Input: dimensioned drawing with shaded views. Units: mm. Origin: part minimum x, y, z. A direction names the side the tool comes from. Give positions to 0.01 mm unless a question says otherwise; leave off trailing zeros. Write each loop counter-clockwise with the first axis right and the second up, starting at its lowest first coordinate (ties: lowest second). Pieces come first, ordered by that corner, then holes.
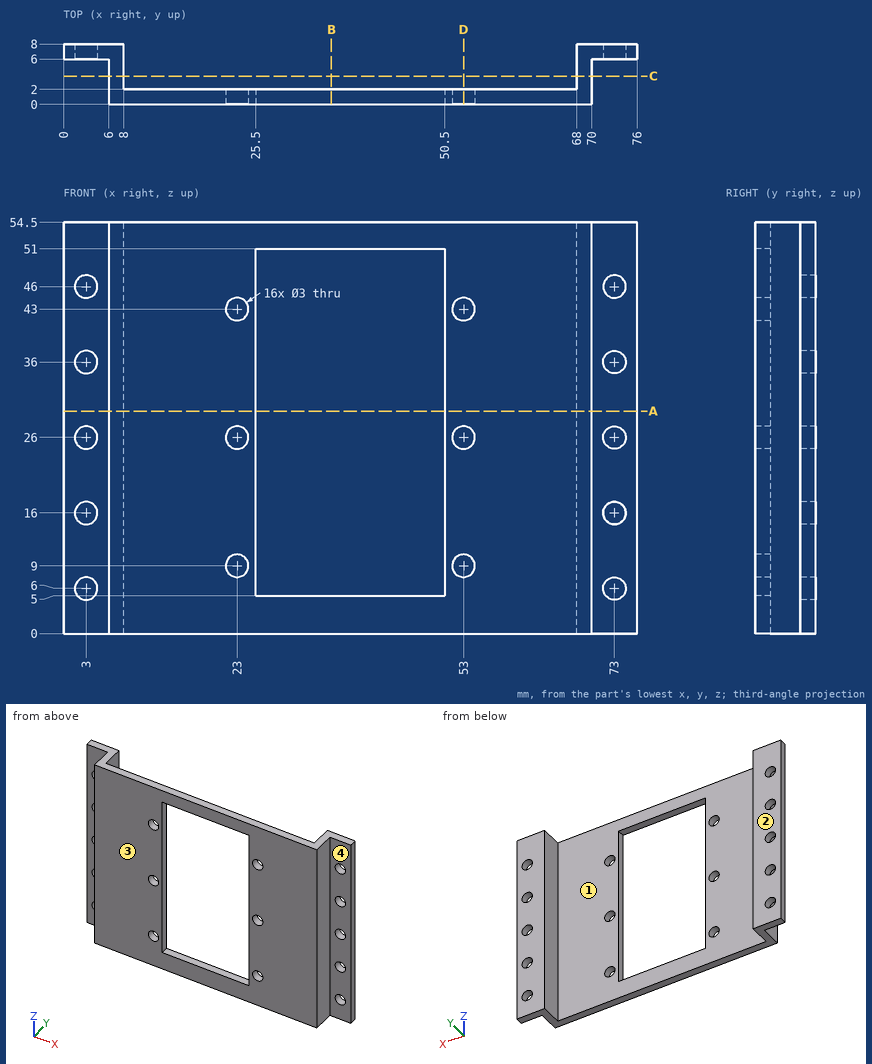
Item 1: Section A-A, the plane z = 29.5. Return the cut outline in (x, y), plus the area to 3 significant figures.
Found:
outline: (0, 6) - (6, 6) - (6, 0) - (25.5, 0) - (25.5, 2) - (8, 2) - (8, 8) - (0, 8) - close; (50.5, 0) - (70, 0) - (70, 6) - (76, 6) - (76, 8) - (68, 8) - (68, 2) - (50.5, 2) - close
area: 126 mm2
Item 2: Section C-C, the plane y = 3.75. Return the cut outline in (x, z).
Found:
outline: (6, 0) - (8, 0) - (8, 54.5) - (6, 54.5) - close; (68, 0) - (70, 0) - (70, 54.5) - (68, 54.5) - close
Item 3: Section B-B, the plane x = 35.5. Return the cut outline in (y, z).
Found:
outline: (0, 0) - (2, 0) - (2, 5) - (0, 5) - close; (0, 51) - (2, 51) - (2, 54.5) - (0, 54.5) - close
Item 4: Section D-D, the plane x = 53. Return the cut outline in (y, z), plus the area to 3 significant figures.
Found:
outline: (0, 0) - (2, 0) - (2, 7.5) - (0, 7.5) - close; (0, 10.5) - (2, 10.5) - (2, 24.5) - (0, 24.5) - close; (0, 27.5) - (2, 27.5) - (2, 41.5) - (0, 41.5) - close; (0, 44.5) - (2, 44.5) - (2, 54.5) - (0, 54.5) - close
area: 91.0 mm2
Item 5: Pin query (flat end, axial travel): pin 1 Ø2 at (y, z) = (5.5, 24) entering from +X; pin 2 Ø5 at (x, z) = (3, 21.5) entering from -Y; pin 3 Ø6 at (x, z) = (61.5, 23) entering from +Y; pin 4 Ø4 at (y, z) = (3, 14.5) entering from +X. Return the tip coordinate at first contact, or that it passes through.
Found:
pin 1: stops at x = 76
pin 2: stops at y = 6
pin 3: stops at y = 2
pin 4: stops at x = 70
Item 6: Line query: L1, parallel to X at y = 6.65, z = 26; L2, parallel to X at y = 4.5, z = 16; L3, parallel to Z at x = 3, y = 7. Output: solid intervals per line, ascending.
Found:
L1: x = 0 to 1.5, 4.5 to 8, 68 to 71.5, 74.5 to 76
L2: x = 6 to 8, 68 to 70
L3: z = 0 to 4.5, 7.5 to 14.5, 17.5 to 24.5, 27.5 to 34.5, 37.5 to 44.5, 47.5 to 54.5
Item 7: Reachability of the marked faces 3 and 4 from +Z, -Z, +X, -X, +Y, -Y: full face, straight path, thin tool, end or side. Return the list, or none.
Found:
face 3: +Z, -Z, +X, -X, -Y
face 4: +Z, -Z, +X, -Y
Item 8: Pull-direction query (X, two-part tool) for the marked faces 1 and 2; classes: +X half, -X half, draft (parallel to the pull), parting line (faces both ways), or undercut.
Found:
face 1: undercut
face 2: draft
